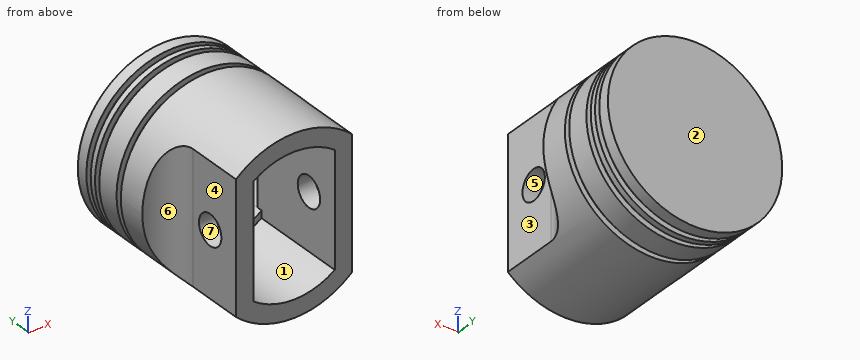
from build123d import *

# Parameters (mm, degrees)
SKETCH1_R               = 15
BOSS_EXTRUDE1_DEPTH     = 30
CUT_EXTRUDE3_DEPTH      = 37.742346142
CUT_EXTRUDE3_DEPTH_BACK = 37.742346142
SKETCH5_W               = 5
SKETCH5_H               = 15
CUT_EXTRUDE5_START      = -10
SKETCH6_R               = 15
CUT_EXTRUDE5_DEPTH      = 10
SKETCH6_4_R             = 14
BOSS_EXTRUDE2_DEPTH     = 10
SKETCH6_5_R             = 15
SKETCH6_5_R_2           = 14
BOSS_EXTRUDE3_DEPTH     = 9
SKETCH6_6_R             = 15
SKETCH6_6_R_2           = 14
CUT_EXTRUDE6_DEPTH      = 5
SKETCH6_7_R             = 15
SKETCH6_7_R_2           = 14
BOSS_EXTRUDE4_DEPTH     = 4
SKETCH6_8_R             = 15
SKETCH6_8_R_2           = 14
CUT_EXTRUDE7_DEPTH      = 3
SKETCH6_9_R             = 15
SKETCH6_9_R_2           = 14
BOSS_EXTRUDE5_DEPTH     = 2
SHELL2_DEPTH            = 27
SHELL2_START            = 18
SHELL2_2_DEPTH          = 9
SHELL2_3_DEPTH          = 17
CUT_EXTRUDE2_DEPTH      = 37.742346142
CUT_EXTRUDE2_DEPTH_BACK = 37.742346142
SKETCH4_R               = 2.6
FILLET1_R               = 5


# Read off the part's stored shape, not the designer's step: Shell2
with BuildPart() as part:
    # Sketch1 → Boss-Extrude1 (new body)
    with BuildSketch(Plane(origin=(0, 0, 0), x_dir=(1, 0, 0), z_dir=(0, 1, 0))):
        with Locations(Location((0, 0, 0), (0, 0, 270))):
            Circle(SKETCH1_R)
    extrude(amount=BOSS_EXTRUDE1_DEPTH)

    # Sketch5 → Cut-Extrude3 (cut, two sides: drawn at the far end of the back side and taken through both)
    with BuildSketch(Plane.XY.offset(-CUT_EXTRUDE3_DEPTH_BACK)):
        with Locations((-12.5, 7.5)):
            Rectangle(SKETCH5_W, SKETCH5_H)
        with Locations((12.5, 7.5)):
            Rectangle(SKETCH5_W, SKETCH5_H)
    extrude(amount=CUT_EXTRUDE3_DEPTH + CUT_EXTRUDE3_DEPTH_BACK, mode=Mode.SUBTRACT)

    # Sketch6 → Cut-Extrude5 (cut)
    with BuildSketch(Plane(origin=(0, 30, 0), x_dir=(1, 0, 0), z_dir=(0, 1, 0)).offset(CUT_EXTRUDE5_START)):
        with Locations(Location((0, 0, 0), (0, 0, 48.189685104))):
            Circle(SKETCH6_R)
    extrude(amount=CUT_EXTRUDE5_DEPTH, mode=Mode.SUBTRACT)

    # Sketch6<4> → Boss-Extrude2 (add)
    with BuildSketch(Plane(origin=(0, 30, 0), x_dir=(1, 0, 0), z_dir=(0, 1, 0))):
        with Locations(Location((0, 0, 0), (0, 0, 270))):
            Circle(SKETCH6_4_R)
    extrude(amount=-BOSS_EXTRUDE2_DEPTH)

    # Sketch6<5> → Boss-Extrude3 (add)
    with BuildSketch(Plane(origin=(0, 30, 0), x_dir=(1, 0, 0), z_dir=(0, 1, 0))):
        with Locations(Location((0, 0, 0), (0, 0, 48.189685104))):
            Circle(SKETCH6_5_R)
        with Locations(Location((0, 0, 0), (0, 0, 270))):
            Circle(SKETCH6_5_R_2, mode=Mode.SUBTRACT)
    extrude(amount=-BOSS_EXTRUDE3_DEPTH)

    # Sketch6<6> → Cut-Extrude6 (cut)
    with BuildSketch(Plane(origin=(0, 30, 0), x_dir=(1, 0, 0), z_dir=(0, 1, 0))):
        with Locations(Location((0, 0, 0), (0, 0, 270))):
            Circle(SKETCH6_6_R)
        with Locations(Location((0, 0, 0), (0, 0, 270))):
            Circle(SKETCH6_6_R_2, mode=Mode.SUBTRACT)
    extrude(amount=-CUT_EXTRUDE6_DEPTH, mode=Mode.SUBTRACT)

    # Sketch6<7> → Boss-Extrude4 (add)
    with BuildSketch(Plane(origin=(0, 30, 0), x_dir=(1, 0, 0), z_dir=(0, 1, 0))):
        with Locations(Location((0, 0, 0), (0, 0, 270))):
            Circle(SKETCH6_7_R)
        with Locations(Location((0, 0, 0), (0, 0, 270))):
            Circle(SKETCH6_7_R_2, mode=Mode.SUBTRACT)
    extrude(amount=-BOSS_EXTRUDE4_DEPTH)

    # Sketch6<8> → Cut-Extrude7 (cut)
    with BuildSketch(Plane(origin=(0, 30, 0), x_dir=(1, 0, 0), z_dir=(0, 1, 0))):
        with Locations(Location((0, 0, 0), (0, 0, 270))):
            Circle(SKETCH6_8_R)
        with Locations(Location((0, 0, 0), (0, 0, 270))):
            Circle(SKETCH6_8_R_2, mode=Mode.SUBTRACT)
    extrude(amount=-CUT_EXTRUDE7_DEPTH, mode=Mode.SUBTRACT)

    # Sketch6<9> → Boss-Extrude5 (add)
    with BuildSketch(Plane(origin=(0, 30, 0), x_dir=(1, 0, 0), z_dir=(0, 1, 0))):
        with Locations(Location((0, 0, 0), (0, 0, 270))):
            Circle(SKETCH6_9_R)
        with Locations(Location((0, 0, 0), (0, 0, 270))):
            Circle(SKETCH6_9_R_2, mode=Mode.SUBTRACT)
    extrude(amount=-BOSS_EXTRUDE5_DEPTH)

    # Shell2 outline → Shell2 (cut)
    with BuildSketch(Plane(origin=(0, 0, 0), x_dir=(1, 0, 0), z_dir=(0, 1, 0))):
        with BuildLine():
            Line((7, -8.485281374), (7, 8.485281374))
            ThreePointArc((7, 8.485281374), (0, 11), (-7, 8.485281374))
            Line((-7, 8.485281374), (-7, -8.485281374))
            ThreePointArc((-7, -8.485281374), (0, -11), (7, -8.485281374))
        make_face()
    extrude(amount=SHELL2_DEPTH, mode=Mode.SUBTRACT)

    # Shell2 2 outline → Shell2 2 (cut)
    with BuildSketch(Plane(origin=(0, 0, 0), x_dir=(1, 0, 0), z_dir=(0, 1, 0)).offset(SHELL2_START)):
        with BuildLine():
            ThreePointArc((7, -8.485281374), (11, 0), (7, 8.485281374))
            Line((7, 8.485281374), (7, -8.485281374))
        make_face()
        with BuildLine():
            Line((-7, -8.485281374), (-7, 8.485281374))
            ThreePointArc((-7, 8.485281374), (-11, 0), (-7, -8.485281374))
        make_face()
    extrude(amount=SHELL2_2_DEPTH, mode=Mode.SUBTRACT)

    # Shell2 3 outline → Shell2 3 (cut)
    with BuildSketch(Plane(origin=(0, 0, 0), x_dir=(1, 0, 0), z_dir=(0, 1, 0))):
        with BuildLine():
            ThreePointArc((-7, 8.485281374), (0, 11), (7, 8.485281374))
            Line((7, 8.485281374), (7, 9.746794345))
            ThreePointArc((7, 9.746794345), (0, 12), (-7, 9.746794345))
            Line((-7, 9.746794345), (-7, 8.485281374))
        make_face()
        with BuildLine():
            Line((7, -9.746794345), (7, -8.485281374))
            ThreePointArc((7, -8.485281374), (0, -11), (-7, -8.485281374))
            Line((-7, -8.485281374), (-7, -9.746794345))
            ThreePointArc((-7, -9.746794345), (0, -12), (7, -9.746794345))
        make_face()
    extrude(amount=SHELL2_3_DEPTH, mode=Mode.SUBTRACT)

    # Sketch4 → Cut-Extrude2 (cut, two sides: drawn at the far end of the back side and taken through both)
    with BuildSketch(Plane(origin=(0, 0, 0), x_dir=(0, 0, -1), z_dir=(1, 0, 0)).offset(-CUT_EXTRUDE2_DEPTH_BACK)):
        with Locations(Location((0, 6, 0), (0, 0, 180))):
            Circle(SKETCH4_R)
    extrude(amount=CUT_EXTRUDE2_DEPTH + CUT_EXTRUDE2_DEPTH_BACK, mode=Mode.SUBTRACT)

    # Fillet1
    fillet1_edges = [part.edges().sort_by_distance(p)[0] for p in [
        (10, 15, 0),
        (-10, 15, 0),
    ]]
    fillet(fillet1_edges, radius=FILLET1_R - 0.0001)  # a hair under: the kernel refuses the full size


solid = part.part
The model under review builds one solid part; all positions refer to its coordinate system, in mm. Face numbers are marked on the shaded views. A direction names the side the tool comes from. Round coordinates to 2 decimals unless told otherwise and drop trailing zeros. Loops run counter-clockwise (first coordinate to the right, second up) from the corner with the lowest first, then second, coordinate; pieces in that order, holes last. Notation, with made-up numbers: M -39.75,54 L -25.75,54 A21 ccw -25.75,65 Z; hole C 59,53 d2. An arc over 180 degrees is marked long. Answer as CSV lines item,"result".
1. Insertion check: pin 1 Ø8 at (y, z) = (5.5, 5) entering from -X; pin 2 Ø9 at (y, z) = (6, 2) entering from +X; pin 3 Ø1.5 at (y, z) = (22.5, -6) entering from +X. Each pin has a flat end and moves straight along its axis. Give the tip position at first contact, or say it passes through.
Outcome:
pin 1,"stops at x = -10"
pin 2,"stops at x = 10.03"
pin 3,"stops at x = 14.05"
2. For the marked faces 1, 2 and 3, list the 3-axis set-ups (+Z, -Z, +X, -X, +Y, -Y) from which the entire face can be reached by the end or side of a thin tool; tool diameter is ignored.
Outcome:
face 1,"-Y"
face 2,"+Z, -Z, +X, -X, +Y"
face 3,"+Z, -Z, +X, -Y"
3. We need section C-C (x = 13). Give the boundary of the cut face in (y, z).
Outcome:
outline,"M 14.58,-7.48 L 20,-7.48 L 20,-5.2 L 21,-5.2 L 21,-7.48 L 25,-7.48 L 25,-5.2 L 26,-5.2 L 26,-7.48 L 27,-7.48 L 27,-5.2 L 28,-5.2 L 28,-7.48 L 30,-7.48 L 30,7.48 L 28,7.48 L 28,5.2 L 27,5.2 L 27,7.48 L 26,7.48 L 26,5.2 L 25,5.2 L 25,7.48 L 21,7.48 L 21,5.2 L 20,5.2 L 20,7.48 L 14.58,7.48 Z"
4. We need section B-B (y = 9.5). Give the boundary of the cut face in (x, z).
Outcome:
outline,"M -10,-11.18 A15 ccw 10,-11.18 L 10,11.18 A15 ccw -10,11.18 Z; hole M -7,-9.75 A12 ccw 7,-9.75 L 7,9.75 A12 ccw -7,9.75 Z"
5. Draft analysis for pull direction Y (two halves, no side actions). For the marked faces 4, 5, 6 and 7, state which applies: pulls with the +Y half, pulls with the -Y half, needs draft (parallel to the pull), parting line crosses it, or undercut.
Outcome:
face 4,"needs draft"
face 5,"undercut"
face 6,"pulls with the -Y half"
face 7,"undercut"
6. We need section A-A (y = 6). Give the boundary of the cut face in (x, z).
Outcome:
outline,"M -10,-11.18 A15 ccw 10,-11.18 L 10,-2.6 L 7,-2.6 L 7,-9.75 A12 cw -7,-9.75 L -7,-2.6 L -10,-2.6 Z; M -10,2.6 L -7,2.6 L -7,9.75 A12 cw 7,9.75 L 7,2.6 L 10,2.6 L 10,11.18 A15 ccw -10,11.18 Z"
7. We need section D-D (y = 16). Give the boundary of the cut face in (x, z), plus the area to 3 significant figures.
Outcome:
outline,"C 0,0 d30; hole M -7,-9.75 A12 ccw 7,-9.75 L 7,9.75 A12 ccw -7,9.75 Z"
area,"391 mm2"
8. To check wall thickness, follow L1, parallel to Y at x = 8.05, z = 0; L2, parallel to Y at x = 8, z = -12; L3, parallel to X at y = 9, z = -3. State the ranges of each line that lie inside material, in increasing order. Write a range as [from, to].
Outcome:
L1,"y = [0, 3.4], [8.6, 18], [27, 30]"
L2,"y = [0, 20], [21, 25], [26, 27], [28, 30]"
L3,"x = [-10, -7], [7, 10]"
